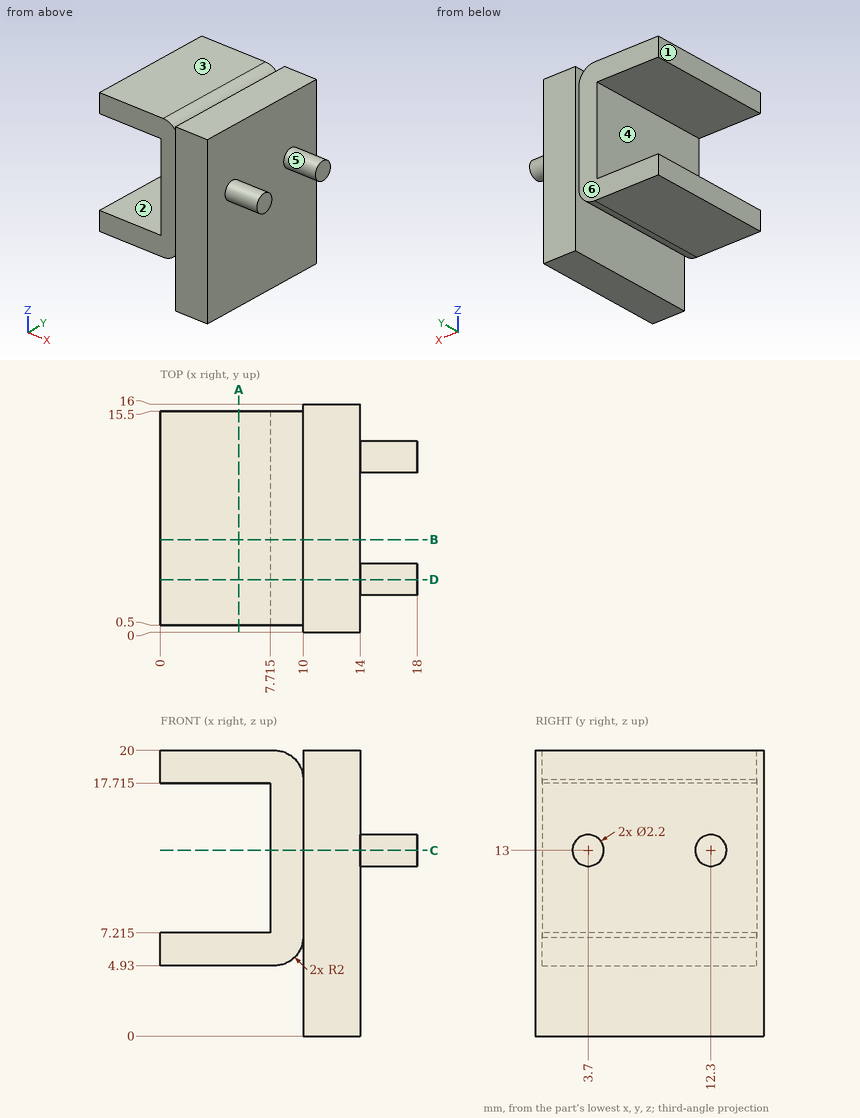
Source: three-view drawing plus pictorial views. Frame: mm from the lowest corner of the part. A direction names the side the tool comes from. Coordinates: 2 decimals unless noted, no trailing zeros. Order: outer loops, then holes, each group sorted by start corner. A loop starts at its lowest first (then second) coordinate and runs counter-clockwise, first axis right, second up. Notation, with made-up numbers: M 78.25,18.5 L 136.25,18.5 A33 cw 136.25,52.5 Z; hole C -6,66.5 d6. An arc over 180 degrees is marked long. Write each question's results on one line, items separated by ' | '. Start each with the question number.
1. Pin query (flat end, axial travel): pin 1 (6 mm diameter, centred on x = 3, z = 10, fed in from +Y); pin 2 (8 mm diameter, centred on y = 9, z = 17.5, fed in from +X); pin 3 (3 mm diameter, centred on y = 11.5, z = 11.5, fed in from -X) (3 decimals). Return the tip coordinate at first contact, or that it passes through.
2. Section B-B, the plane y = 6.5. Return the cut outline in (x, z) (3 decimals).
3. Material intervals for L1, parallel to Z at x = 7.5, y = 9.5 (3 decimals); L2, parallel to X at y = 8.75, z = 1.25; L3, parallel to X at y = 15, z = 11.25 (3 decimals), sorted ascending.
4. Section A-A, the plane x = 5.5. Return the cut outline in (y, z) (3 decimals), then the cut area to 4 significant figures.
5. Section D-D, the plane y = 3.7. Return the cut outline in (x, z) (3 decimals).
6. Reachability of the marked faces 4, 5 and 6 from +Z, -Z, +X, -X, +Y, -Y: full face, straight path, thin tool, end or side. Return the list, or none.
7. Section C-C, the plane z = 13. Return the cut outline in (x, y) (3 decimals).
8. Draft query along Z for the marked faces 1, 2 and 3. Return one class per face: +Z half, -Z half, draft (parallel to the pull), parting line (faces both ways), or undercut.
Solution:
1) pin 1: y = 15.5 | pin 2: x = 14 | pin 3: x = 7.715
2) outline: M 0,4.93 L 8,4.93 A2 ccw 10,6.93 L 10,0 L 14,0 L 14,20 L 10,20 L 10,18 A2 ccw 8,20 L 0,20 L 0,17.715 L 7.715,17.715 L 7.715,7.215 L 0,7.215 Z
3) L1: 4.93 to 7.215, 17.715 to 20 | L2: 10 to 14 | L3: 7.715 to 14
4) outline: M 0.5,4.93 L 15.5,4.93 L 15.5,7.215 L 0.5,7.215 Z; M 0.5,17.715 L 15.5,17.715 L 15.5,20 L 0.5,20 Z | area: 68.55 mm²
5) outline: M 0,4.93 L 8,4.93 A2 ccw 10,6.93 L 10,0 L 14,0 L 14,11.9 L 18,11.9 L 18,14.1 L 14,14.1 L 14,20 L 10,20 L 10,18 A2 ccw 8,20 L 0,20 L 0,17.715 L 7.715,17.715 L 7.715,7.215 L 0,7.215 Z
6) face 4: -X, +Y, -Y | face 5: +X | face 6: +Z, -Z, -X, +Y
7) outline: M 7.715,0.5 L 10,0.5 L 10,0 L 14,0 L 14,2.6 L 18,2.6 L 18,4.8 L 14,4.8 L 14,11.2 L 18,11.2 L 18,13.4 L 14,13.4 L 14,16 L 10,16 L 10,15.5 L 7.715,15.5 Z
8) face 1: draft | face 2: undercut | face 3: +Z half
